Can you work these out from the model? Positions are in its coordinate system, mm. Face numbers are marked on the shaded views. Give positions to 0.01 mm unless a question says otherwise; leave off trailing zeros. Loops run counter-clockwise (first coordinate to the right, second up) from the corner with the lowest first, then second, coordinate; pieces in that order, holes last. Notation, with made-up numbers: M -21.5,71.25 L 0.5,71.25 A30 ccw 0.5,106.25 Z; hole C 46,-34 d8. An arc over 180 degrees is marked long. Answer as a JSON object with one key per item and string values.
```python
from build123d import *

# Parameters (mm, degrees)
SKETCH1_R                 = 7.9375
SKETCH1_R_2               = 6.35
BOSS_EXTRUDE1_DEPTH       = 76.2
BOSS_EXTRUDE2_START       = -3.175
SKETCH2_R                 = 15.875
SKETCH2_R_2               = 6.35
BOSS_EXTRUDE2_DEPTH       = 3.175
F_4_CLEARANCE_HOLE1_D     = 2.9464
F_4_CLEARANCE_HOLE1_DEPTH = 4
F_4_CLEARANCE_HOLE1_TIP   = 0.885187864
CUT_EXTRUDE1_DEPTH        = 80.43847462
CUT_EXTRUDE1_DEPTH_BACK   = 80.43847462
SKETCH6_W                 = 4.137147463
SKETCH6_H                 = 15


with BuildPart() as part:
    # Sketch1 → Boss-Extrude1 (new body)
    with BuildSketch(Plane.XY):
        with Locations(Location((0, 0, 0), (0, 0, 180))):
            Circle(SKETCH1_R)
        with Locations(Location((0, 0, 0), (0, 0, 180))):
            Circle(SKETCH1_R_2, mode=Mode.SUBTRACT)
    extrude(amount=BOSS_EXTRUDE1_DEPTH)

    # Sketch2 → Boss-Extrude2 (add)
    with BuildSketch(Plane.XY.offset(76.2).offset(BOSS_EXTRUDE2_START)):
        Circle(SKETCH2_R)
        with Locations(Location((0, 0, 0), (0, 0, 180))):
            Circle(SKETCH2_R_2, mode=Mode.SUBTRACT)
    extrude(amount=BOSS_EXTRUDE2_DEPTH)

    # #4 Clearance Hole1
    with Locations(Plane.XY.offset(76.2)):
        with Locations((0, 12.7), (0, -12.7), (12.7, 0), (-12.7, 0)):
            Hole(F_4_CLEARANCE_HOLE1_D / 2, depth=F_4_CLEARANCE_HOLE1_DEPTH)
            with Locations((0, 0, -(F_4_CLEARANCE_HOLE1_DEPTH + F_4_CLEARANCE_HOLE1_TIP / 2))):  # 118° drill point
                Cone(0, F_4_CLEARANCE_HOLE1_D / 2, F_4_CLEARANCE_HOLE1_TIP, mode=Mode.SUBTRACT)

    # Sketch6 → Cut-Extrude1 (cut, two sides: drawn at the far end of the back side and taken through both)
    with BuildSketch(Plane(origin=(0, 0, 0), x_dir=(1, 0, 0), z_dir=(0, 1, 0)).offset(-CUT_EXTRUDE1_DEPTH_BACK)):
        with Locations((9.506073732, -7.5)):
            Rectangle(SKETCH6_W, SKETCH6_H)
    extrude(amount=CUT_EXTRUDE1_DEPTH + CUT_EXTRUDE1_DEPTH_BACK, mode=Mode.SUBTRACT)


solid = part.part
```
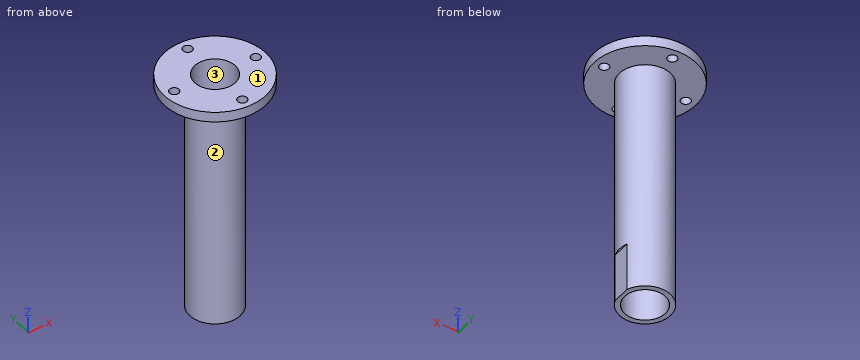
1) Suppose I cut it at A-A, the plane x = 0. Give the number of separate pieces and of enclosed holes in the cut face, and give its area (3 significant figures).
Answer list:
{"separate pieces": "4", "enclosed holes": "0", "area": "274 mm^2"}
2) Please list where these lines run through material, in increasing order: line 1 along Y through (x, z) = (0, 18); line 2 along Z through (x, y) = (12.5, 3) (3 decimals); line 3 along Y through (x, z) = (5, 36). Write a range as from..to.
Answer list:
{"line 1": "-7.94..-6.35, 6.35..7.94", "line 2": "73.025..76.2", "line 3": "-6.16..-3.91, 3.91..6.16"}
3) Will these pins go through, and if not, where does the flat tip stop? pin 1 Ø8 at (x, z) = (3.5, 15) entering from -Y; pin 2 Ø6 at (y, z) = (5, 36.5) entering from -X; pin 3 Ø2.5 at (x, y) = (0, 12.7) entering from +Z; pin 4 Ø8 at (x, z) = (5.5, 32.5) entering from -Y.
Answer list:
{"pin 1": "y = -7.94", "pin 2": "x = -7.68", "pin 3": "through", "pin 4": "y = -7.79"}
4) Suppose I cut it at D-D, the plane x = -13. Write out the boundary of the cut face in (y, z) (3 decimals).
Answer list:
{"outline": "M -9.111,73.025 L -1.442,73.025 L -1.442,76.2 L -9.111,76.2 Z; M 1.442,73.025 L 9.111,73.025 L 9.111,76.2 L 1.442,76.2 Z"}
5) If we mould it in two halves opening along X, with no side actions, what happens to the marked faces 1, 2 and 3? For each: +X half, -X half, draft (parallel to the pull), parting line (faces both ways), or undercut.
Answer list:
{"face 1": "draft", "face 2": "parting line", "face 3": "undercut"}
